Study the drawing (mm; zero at the part's minimum x, y, z) and answer. Coordinates: 2 decimals unless noted, no trailing zeros. Write each loop counter-clockwise with the first axis right and the second up, starting at its lowest first coordinate (ties: lowest second). Pieces come first, ordered by that corner, then holes. Notation, with made-up numbers: (-36, 12) - (-11, 12) arc R26 cw to (-11, 42) - close; hole circle Ø4 at (88, 65.5). An arc over 180 degrees is marked (long way). One line per item, written item: value.
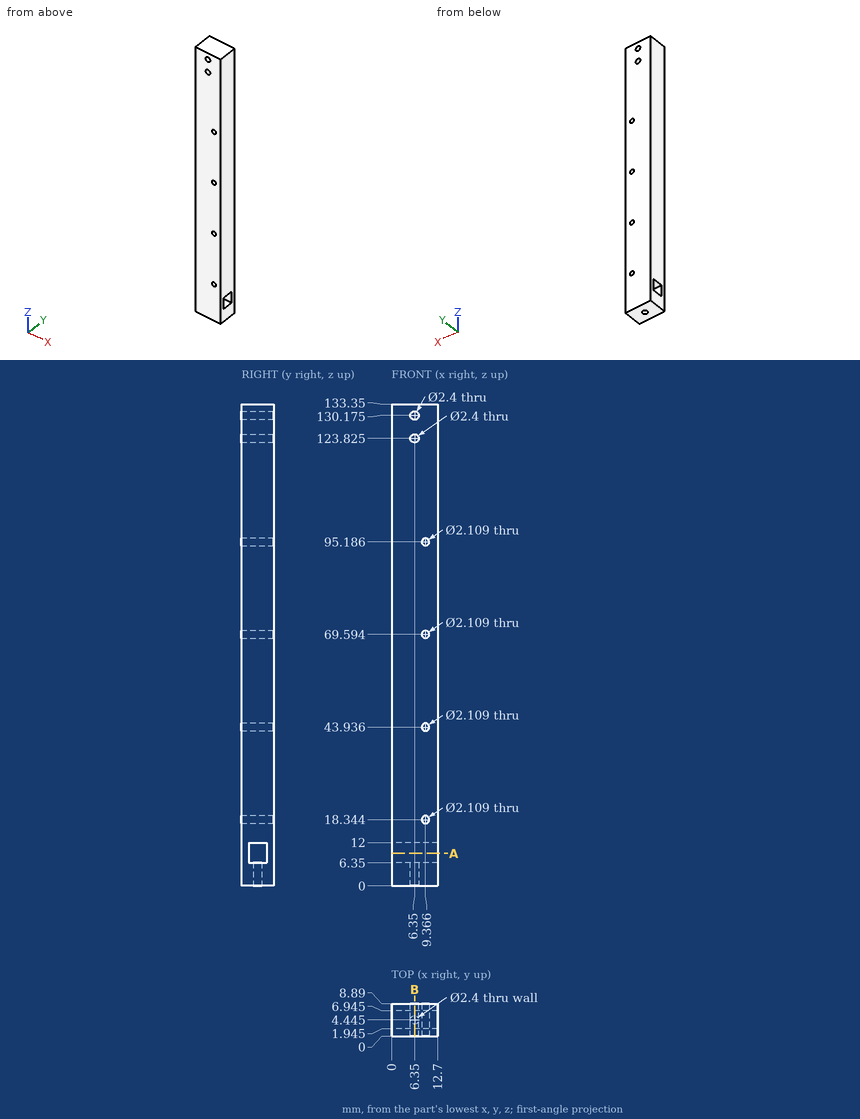
Item 1: Section B-B, the plane x = 6.35 is taken. Give the number of separate pieces and of enclosed holes in the cut face, then the cut area to 3 significant figures.
Evaluation:
separate pieces: 3
enclosed holes: 0
area: 1,100 mm2
Item 2: Section A-A, the plane z = 9 is taken. Determine the outline of the cut face in (x, y) (1 decimal).
Evaluation:
outline: (0, 0) - (12.7, 0) - (12.7, 1.9) - (0, 1.9) - close; (0, 6.9) - (12.7, 6.9) - (12.7, 8.9) - (0, 8.9) - close
Item 3: Consider probe 1 along Y at (x, z) = (11.5, 8) (1 decimal); probe 2 along X at (y, z) = (6.5, 18.5); probe 3 along Z at (x, y) = (11.25, 6.5). Determine where each line is inside the solid, lowest interval first.
Evaluation:
probe 1: y = 0 to 1.9, 6.9 to 8.9
probe 2: x = 0 to 8.32, 10.41 to 12.7
probe 3: z = 0 to 6.35, 12 to 133.35
